```python
from build123d import *

# Parameters (mm, degrees)
F0_R     = 2.75
F0_R_2   = 1.5
F1_DEPTH = 4
F2_DEPTH = 17
F4_DEPTH = 25


with BuildPart() as f1:
    # F0 (on Top) → F1 (new body)
    with BuildSketch(Plane.XY):
        Polygon((-6.25, -20.25), (6.25, -20.25), (6.25, -9.8827272505), (-3.125, -9.8827272505), (-6.25, -13.25), align=None)
        with BuildLine():
            ThreePointArc((-2.4743686063, -14.3), (0, -12.75), (2.4743686063, -14.3))
            Line((2.4743686063, -14.3), (2.9, -14.3))
            Line((2.9, -14.3), (2.9, -16.7))
            Line((2.9, -16.7), (2.4743686063, -16.7))
            ThreePointArc((2.4743686063, -16.7), (0, -18.25), (-2.4743686063, -16.7))
            Line((-2.4743686063, -16.7), (-2.9, -16.7))
            Line((-2.9, -16.7), (-2.9, -14.3))
            Line((-2.9, -14.3), (-2.4743686063, -14.3))
        make_face(mode=Mode.SUBTRACT)
        Polygon((-3.125, -9.8827272505), (6.25, -9.8827272505), (6.25, -6.5154545009), (0, -6.5154545009), align=None)
        Polygon((0, -6.5154545009), (6.25, -6.5154545009), (6.25, 20.25), (-6.25, 20.25), (-6.25, 13.25), (0, 6.5154545009), (0, 0), align=None)
        with Locations((0, 15.5)):
            Circle(F0_R, mode=Mode.SUBTRACT)
        with Locations((0, 15.5)):
            Circle(F0_R)
        with Locations((0, 15.5)):
            Circle(F0_R_2, mode=Mode.SUBTRACT)
        with BuildLine():
            ThreePointArc((-0.9, -14.3), (0, -14), (0.9, -14.3))
            Line((0.9, -14.3), (2.4743686063, -14.3))
            ThreePointArc((2.4743686063, -14.3), (0, -12.75), (-2.4743686063, -14.3))
            Line((-2.4743686063, -14.3), (-0.9, -14.3))
        make_face()
        with BuildLine():
            ThreePointArc((-0.9, -16.7), (-1.5, -15.5), (-0.9, -14.3))
            Line((-0.9, -14.3), (-2.4743686063, -14.3))
            ThreePointArc((-2.4743686063, -14.3), (-2.75, -15.5), (-2.4743686063, -16.7))
            Line((-2.4743686063, -16.7), (-0.9, -16.7))
        make_face()
        with BuildLine():
            Line((2.4743686063, -16.7), (0.9, -16.7))
            ThreePointArc((0.9, -16.7), (0, -17), (-0.9, -16.7))
            Line((-0.9, -16.7), (-2.4743686063, -16.7))
            ThreePointArc((-2.4743686063, -16.7), (0, -18.25), (2.4743686063, -16.7))
        make_face()
        with BuildLine():
            ThreePointArc((0.9, -14.3), (1.3416407865, -14.8291796068), (1.5, -15.5))
            ThreePointArc((1.5, -15.5), (1.3416407865, -16.1708203932), (0.9, -16.7))
            Line((0.9, -16.7), (2.4743686063, -16.7))
            ThreePointArc((2.4743686063, -16.7), (2.6802064909, -16.1156242087), (2.75, -15.5))
            ThreePointArc((2.75, -15.5), (2.6802064909, -14.8843757913), (2.4743686063, -14.3))
            Line((2.4743686063, -14.3), (0.9, -14.3))
        make_face()
        with BuildLine():
            ThreePointArc((-2.4743686063, -16.7), (-2.75, -15.5), (-2.4743686063, -14.3))
            Line((-2.4743686063, -14.3), (-2.9, -14.3))
            Line((-2.9, -14.3), (-2.9, -16.7))
            Line((-2.9, -16.7), (-2.4743686063, -16.7))
        make_face()
        with BuildLine():
            Line((2.9, -14.3), (2.4743686063, -14.3))
            ThreePointArc((2.4743686063, -14.3), (2.6802064909, -14.8843757913), (2.75, -15.5))
            ThreePointArc((2.75, -15.5), (2.6802064909, -16.1156242087), (2.4743686063, -16.7))
            Line((2.4743686063, -16.7), (2.9, -16.7))
            Line((2.9, -16.7), (2.9, -14.3))
        make_face()
    extrude(amount=F1_DEPTH)

    # F0 (on Top) → F2 (join)
    with BuildSketch(Plane.XY):
        Polygon((-6.25, -20.25), (6.25, -20.25), (6.25, -9.8827272505), (-3.125, -9.8827272505), (-6.25, -13.25), align=None)
        with BuildLine():
            ThreePointArc((-2.4743686063, -14.3), (0, -12.75), (2.4743686063, -14.3))
            Line((2.4743686063, -14.3), (2.9, -14.3))
            Line((2.9, -14.3), (2.9, -16.7))
            Line((2.9, -16.7), (2.4743686063, -16.7))
            ThreePointArc((2.4743686063, -16.7), (0, -18.25), (-2.4743686063, -16.7))
            Line((-2.4743686063, -16.7), (-2.9, -16.7))
            Line((-2.9, -16.7), (-2.9, -14.3))
            Line((-2.9, -14.3), (-2.4743686063, -14.3))
        make_face(mode=Mode.SUBTRACT)
    extrude(amount=F2_DEPTH)

    # F3 (on Front) → F4 (cut)
    with BuildSketch(Plane.XZ):
        with BuildLine():
            ThreePointArc((0, 9), (1.0606601718, 9.4393398282), (1.5, 10.5))
            ThreePointArc((1.5, 10.5), (-1.0606601718, 11.5606601718), (0, 9))
        make_face()
    extrude(amount=F4_DEPTH, mode=Mode.SUBTRACT)


solid = f1.part
```
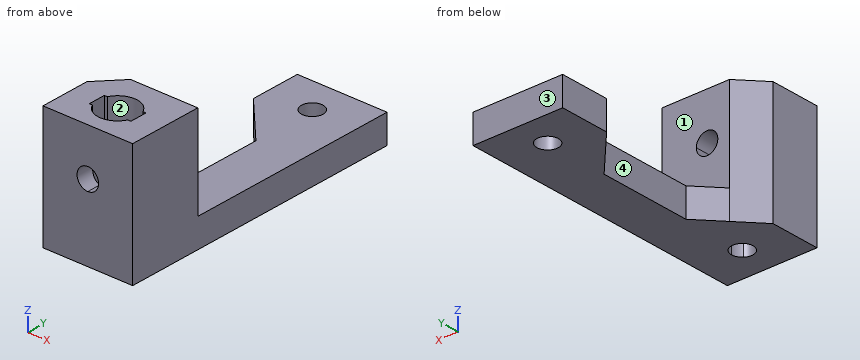
Geometry: final body of the model. Coordinates: model frame, mm. Face numbers are marked on the shaded views. A direction names the side the tool comes from. Give positions to 0.01 mm unless a question says otherwise; leave off trailing zeros. Order: outer loops, then holes, each group sorted by start corner. A loop starts at its lowest first (then second) coordinate and runs counter-clockwise, first axis right, second up. Notation, with made-up numbers: M 86,49.25 L 123,49.25 A26 ccw 123,76.25 Z; hole C 65,-19.5 d7. An arc over 180 degrees is marked long. Answer as CSV lines item,"result". Start each with the question number.
1) First-contact query: P1, Ø2.5, axis at x = 0, y = -15.5, coming from the -Z side; P2, Ø6, axis at x = -1, y = 1, coming from the +Z side; P3, Ø3, axis at x = 2, z = 10.5, coming from the +Y side; P4, Ø1.2, axis at y = 0, z = 2.5, coming from the -X side. Flat tips, straight axial feed; report the tip coordinate or a pass-through.
2) Cut plane D-D (x = 4.5). Output: boundary loops of the cut face in (y, z), then the cut area to 3 significant figures.
3) Line query: line 1 (X direction, y = -15.5, z = 2.35); line 2 (Y direction, x = -0.75, z = 1); line 3 (Z direction, x = 2, y = 1). Output: solid intervals per line, ascending. Write a range as from..to.
4) Cut plane B-B (z = 14). Output: boundary loops of the cut face in (x, y) (3 decimals), then the cut area to 3 significant figures.
5) Cut plane A-A (y = 15.5). Output: boundary loops of the cut face in (x, z).
6) Set-up query: the marked faces 1, 2, 3 and 4. Return all of +Z, -Z, +X, -X, +Y, -Y with unobstructed straight access to the full face (end or side cutting, diameter ignored); none if empty.
7) Cut plane C-C (x = -4). Output: boundary loops of the cut face in (y, z).
Findings below:
1,P1,"passes through"
1,P2,"stops at z = 4"
1,P3,"stops at y = -9.88"
1,P4,"stops at x = 0"
2,outline,"M -20.25,0 L 20.25,0 L 20.25,4 L -9.88,4 L -9.88,17 L -20.25,17 Z"
2,area,"297 mm²"
3,line 1,"x = -6.25..-1.5, 1.5..6.25"
3,line 2,"y = -20.25..-16.8, -14.2..-7.32, 7.32..14.2, 16.8..20.25"
3,line 3,"z = 0..4"
4,outline,"M -6.25,-20.25 L 6.25,-20.25 L 6.25,-9.883 L -3.125,-9.883 L -6.25,-13.25 Z; hole M -2.9,-16.7 L -2.474,-16.7 A2.75 ccw 2.474,-16.7 L 2.9,-16.7 L 2.9,-14.3 L 2.474,-14.3 A2.75 ccw -2.474,-14.3 L -2.9,-14.3 Z"
4,area,"99.4 mm²"
5,outline,"M -6.25,0 L -1.5,0 L -1.5,4 L -6.25,4 Z; M 1.5,0 L 6.25,0 L 6.25,4 L 1.5,4 Z"
6,face 1,"+Z, +X, -X, +Y"
6,face 2,"+Z"
6,face 3,"+Z, -Z, +X, -X, +Y"
6,face 4,"+Z, -Z, -X"
7,outline,"M -20.25,0 L -10.83,0 L -10.83,17 L -20.25,17 Z; M 10.83,0 L 20.25,0 L 20.25,4 L 10.83,4 Z"
